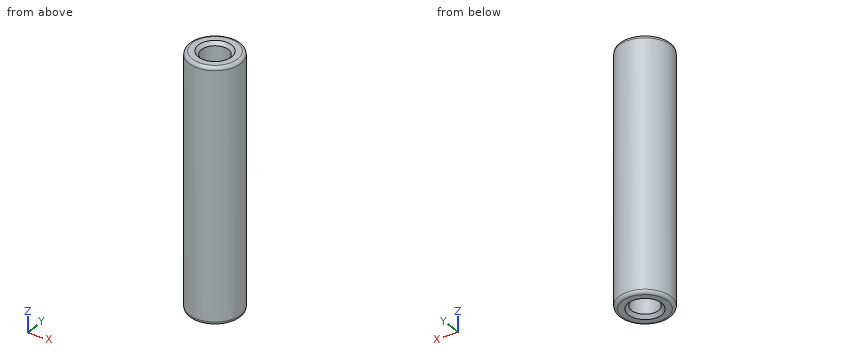
from build123d import *

# Parameters (mm, degrees)
F0_R     = 12.7
F0_R_2   = 6.604
F1_DEPTH = 123.03252
F2_SIZE  = 1.5875
F3_R     = 1.5875


with BuildPart() as f1:
    # F0 (on Top) → F1 (new body)
    with BuildSketch(Plane.XY):
        Circle(F0_R)
        Circle(F0_R_2, mode=Mode.SUBTRACT)
    extrude(amount=F1_DEPTH)

    # F2
    f2_edges = [f1.edges().sort_by_distance(p)[0] for p in [
        (6.604, 0, 61.51626),
        (-6.604, 0, 0),
        (-6.604, 0, 123.03252),
    ]]
    chamfer(f2_edges, length=F2_SIZE)

    # F3
    f3_edges = [f1.edges().sort_by_distance(p)[0] for p in [
        (12.7, 0, 61.51626),
        (-12.7, 0, 0),
        (-12.7, 0, 123.03252),
    ]]
    fillet(f3_edges, radius=F3_R)


solid = f1.part
Read the model definition and answer for the solid it produces. Units are mm, in the model's axes. Coordinates: 2 decimals unless noted, no trailing zeros. Order: outer loops, then holes, each group sorted by start corner. A loop starts at its lowest first (then second) coordinate and runs counter-clockwise, first axis right, second up. Notation, with made-up numbers: (60.5, 2.5) -> (90.5, 2.5) arc R15 cw to (90.5, 8.5) -> close; hole circle Ø9 at (21.5, 1.5). An arc over 180 degrees is marked (long way). Answer as a JSON object with one key per item and string values.
1) Consider line 1 along Y through (x, z) = (0, 57); line 2 along X through (y, z) = (-3.25, 104.5); line 3 along X through (y, z) = (2.75, 88). Determine where each line is inside the solid, lowest interval first. Write a range as from..to.
Model answer:
{"line 1": "y = -12.7..-6.6, 6.6..12.7", "line 2": "x = -12.28..-5.75, 5.75..12.28", "line 3": "x = -12.4..-6, 6..12.4"}
2) A cutting plane is placed at A-A, the plane y = 0. Determine the outline of the cut face in (x, z) (1 decimal), plus the area to 3 significant figures.
Model answer:
{"outline": "(-12.7, 1.6) arc R1.6 ccw to (-11.1, 0) -> (-8.2, 0) -> (-6.6, 1.6) -> (-6.6, 121.4) -> (-8.2, 123) -> (-11.1, 123) arc R1.6 ccw to (-12.7, 121.4) -> close; (6.6, 1.6) -> (8.2, 0) -> (11.1, 0) arc R1.6 ccw to (12.7, 1.6) -> (12.7, 121.4) arc R1.6 ccw to (11.1, 123) -> (8.2, 123) -> (6.6, 121.4) -> close", "area": "1,490 mm²"}
3) A cutting plane is placed at C-C, the plane z = 109.5. Determine the outline of the cut face in (x, y), plus the area to 3 significant figures.
Model answer:
{"outline": "circle Ø25.4 at (0, 0); hole circle Ø13.21 at (0, 0)", "area": "370 mm²"}
4) Each of these flat-tipped pins is pushed along its axis until it touches: pin 1 (3 mm diameter, centred on x = 9.5, z = 82, fed in from +Y); pin 2 (15 mm diameter, centred on x = 0, y = 0, fed in from -Z); pin 3 (4 mm diameter, centred on x = 9, z = 61.5, fed in from +Y). Where does it stop, or does it pass through?
Model answer:
{"pin 1": "stops at y = 9.86", "pin 2": "stops at z = 0.69", "pin 3": "stops at y = 10.6"}
